The listing builds one solid part. Answer for the finished solid, in the listing's coordinates (mm). Coordinates: 2 decimals unless noted, no trailing zeros. Loops run counter-clockwise (first coordinate to the right, second up) from the corner with the lowest first, then second, coordinate; pieces in that order, holes last. Notation, with made-up numbers: (58, 81.5) -> (73, 81.5) arc R26 cw to (73, 107.5) -> close; hole circle Ø8 at (78, 74). An arc over 180 degrees is marked (long way). Answer in a Markdown table with one row per item.
```python
from build123d import *

# Parameters (mm, degrees)
SKETCH1_W           = 80
SKETCH1_H           = 80
SKETCH1_R           = 2
SKETCH1_R_2         = 1.75
BOSS_EXTRUDE1_DEPTH = 4
CUT_EXTRUDE2_DEPTH  = 57.709787515
FILLET1_R           = 10
FILLET2_R           = 20
BOSS_EXTRUDE3_DEPTH = 4
SKETCH6_R           = 1.75
CUT_EXTRUDE3_DEPTH  = 4
SKETCH7_R           = 1.5
CUT_EXTRUDE4_DEPTH  = 10
CHAMFER1_SIZE       = 8
CHAMFER1_SIZE2      = 11.425184054
SKETCH8_W           = 10
SKETCH8_H           = 34
BOSS_EXTRUDE4_DEPTH = 4
SKETCH9_R           = 2
CUT_EXTRUDE5_DEPTH  = 4
CHAMFER2_SIZE       = 10
CHAMFER2_SIZE2      = 8.390996312


with BuildPart() as part:
    # Sketch1 → Boss-Extrude1 (new body)
    with BuildSketch(Plane(origin=(0, 0, 0), x_dir=(1, 0, 0), z_dir=(0, 1, 0))):
        Rectangle(SKETCH1_W, SKETCH1_H)
        with Locations(Location((-24.748737342, 24.748737342, 0), (0, 0, 270))):
            Circle(SKETCH1_R, mode=Mode.SUBTRACT)
        with Locations(Location((24.748737342, 24.748737342, 0), (0, 0, 270))):
            Circle(SKETCH1_R, mode=Mode.SUBTRACT)
        with Locations(Location((24.748737342, -24.748737342, 0), (0, 0, 270))):
            Circle(SKETCH1_R, mode=Mode.SUBTRACT)
        with Locations(Location((-24.748737342, -24.748737342, 0), (0, 0, 270))):
            Circle(SKETCH1_R, mode=Mode.SUBTRACT)
        with Locations(Location((-10, 10, 0), (0, 0, 270))):
            Circle(SKETCH1_R_2, mode=Mode.SUBTRACT)
        with Locations(Location((10, 10, 0), (0, 0, 270))):
            Circle(SKETCH1_R_2, mode=Mode.SUBTRACT)
        with Locations(Location((10, -10, 0), (0, 0, 270))):
            Circle(SKETCH1_R_2, mode=Mode.SUBTRACT)
        with Locations(Location((-10, -10, 0), (0, 0, 270))):
            Circle(SKETCH1_R_2, mode=Mode.SUBTRACT)
        with Locations(Location((31.819805153, 31.819805153, 0), (0, 0, 270))):
            Circle(SKETCH1_R, mode=Mode.SUBTRACT)
        with Locations(Location((-31.819805153, 31.819805153, 0), (0, 0, 270))):
            Circle(SKETCH1_R, mode=Mode.SUBTRACT)
        with Locations(Location((-31.819805153, -31.819805153, 0), (0, 0, 270))):
            Circle(SKETCH1_R, mode=Mode.SUBTRACT)
        with Locations(Location((31.819805153, -31.819805153, 0), (0, 0, 270))):
            Circle(SKETCH1_R, mode=Mode.SUBTRACT)
    extrude(amount=BOSS_EXTRUDE1_DEPTH)

    # Sketch2 → Cut-Extrude2 (cut, through all)
    with BuildSketch(Plane(origin=(0, 4, 0), x_dir=(1, 0, 0), z_dir=(0, 1, 0))):
        Polygon((-40, 30), (-40, -30), (-17, -10), (-17, 10), align=None)
        Polygon((30, 40), (-30, 40), (-10, 17), (10, 17), align=None)
        Polygon((40, -30), (40, 30), (17, 10), (17, -10), align=None)
        Polygon((-30, -40), (30, -40), (10, -17), (-10, -17), align=None)
    extrude(amount=-CUT_EXTRUDE2_DEPTH, mode=Mode.SUBTRACT)

    # Fillet1
    # the kernel refuses this fillet: 10 mm, written as the material it takes off along each edge
    with BuildSketch(Plane(origin=(-30, 15.390762292, 40), x_dir=(-1, 0, 0), z_dir=(0, -1, 0)), Plane(origin=(-40, 15.390762292, 30), x_dir=(0.754605522163505, 0, -0.6561787149247863), z_dir=(0, -1, 0)), Plane(origin=(-40, 15.390762292, -30), x_dir=(0, 0, -1), z_dir=(0, -1, 0)), Plane(origin=(-30, 15.390762292, -40), x_dir=(0.6561787149247871, 0, 0.7546055221635043), z_dir=(0, -1, 0)), Plane(origin=(30, 15.390762292, -40), x_dir=(1, 0, 0), z_dir=(0, -1, 0)), Plane(origin=(40, 15.390762292, -30), x_dir=(-0.7546055221635045, 0, 0.6561787149247867), z_dir=(0, -1, 0)), Plane(origin=(40, 15.390762292, 30), x_dir=(0, 0, 1), z_dir=(0, -1, 0))) as fillet1_piece_1:
        with BuildLine():
            CenterArc((FILLET1_R * 0.455630491663, FILLET1_R), FILLET1_R, 221.009086902, 48.990913098)
            Line((-FILLET1_R * 0.2989750305, FILLET1_R * 0.343821285075), (0, 0))
            Line((0, 0), (FILLET1_R * 0.455630491663, 0))
        make_face()
    extrude(amount=26.781524583, mode=Mode.SUBTRACT)
    with BuildSketch(Plane(origin=(-40, -25, 40), x_dir=(0, 0, -1), z_dir=(0, 1, 0)), Plane(origin=(-40, -25, -40), x_dir=(1, 0, 0), z_dir=(0, 1, 0)), Plane(origin=(40, -25, -40), x_dir=(0, 0, 1), z_dir=(0, 1, 0)), Plane(origin=(40, -25, 40), x_dir=(-1, 0, 0), z_dir=(0, 1, 0))) as fillet1_piece_2:
        with BuildLine():
            CenterArc((FILLET1_R, -FILLET1_R), FILLET1_R, 90, 90)
            Line((0, -FILLET1_R), (0, 0))
            Line((0, 0), (FILLET1_R, 0))
        make_face()
    extrude(amount=54, mode=Mode.SUBTRACT)
    with BuildSketch(Plane(origin=(30, 15.390762292, 40), x_dir=(1, 0, 0), z_dir=(0, -1, 0))) as fillet1_piece_3:
        with BuildLine():
            CenterArc((FILLET1_R * 0.455630491663, -FILLET1_R), FILLET1_R, 90, 48.990913098)
            Line((-FILLET1_R * 0.2989750305, -FILLET1_R * 0.343821285075), (0, 0))
            Line((0, 0), (FILLET1_R * 0.455630491663, 0))
        make_face()
    extrude(amount=26.781524583, mode=Mode.SUBTRACT)

    # Fillet2
    fillet2_edges = [part.edges().sort_by_distance(p)[0] for p in [
        (10, 2, 17),
        (-10, 2, 17),
        (-17, 2, 10),
        (-17, 2, -10),
        (17, 2, -10),
        (17, 2, 10),
        (-10, 2, -17),
        (10, 2, -17),
    ]]
    fillet(fillet2_edges, radius=FILLET2_R)

    # Sketch5 → Boss-Extrude3 (add)
    with BuildSketch(Plane(origin=(0, 4, 0), x_dir=(1, 0, 0), z_dir=(0, 1, 0))):
        Polygon((-0.887390167, 17), (13.289046487, 12.123524967), (13.289046487, -13.496190448), (-0.887390167, -17), (59.112609833, -17), (59.112609833, 17), align=None)
    boss_extrude3 = extrude(amount=-BOSS_EXTRUDE3_DEPTH)

    # Sketch6 → Cut-Extrude3 (cut)
    with BuildSketch(Plane(origin=(0, 4, 0), x_dir=(1, 0, 0), z_dir=(0, 1, 0))):
        with Locations(Location((25, 10, 0), (0, 0, 270))):
            Circle(SKETCH6_R)
        with Locations(Location((45, 10, 0), (0, 0, 270))):
            Circle(SKETCH6_R)
        with Locations(Location((25, -10, 0), (0, 0, 270))):
            Circle(SKETCH6_R)
        with Locations(Location((45, -10, 0), (0, 0, 270))):
            Circle(SKETCH6_R)
    cut_extrude3 = extrude(amount=-CUT_EXTRUDE3_DEPTH, mode=Mode.SUBTRACT)

    # Mirror1: Boss-Extrude3, Cut-Extrude3 across plane
    add(boss_extrude3.mirror(Plane(origin=(0, 0, 0), x_dir=(0, 0, 1), z_dir=(1, 0, 0))))
    add(cut_extrude3.mirror(Plane(origin=(0, 0, 0), x_dir=(0, 0, 1), z_dir=(1, 0, 0))), mode=Mode.SUBTRACT)

    # Sketch7 → Cut-Extrude4 (cut)
    with BuildSketch(Plane(origin=(0, 4, 0), x_dir=(1, 0, 0), z_dir=(0, 1, 0))):
        with Locations(Location((55, 7.25, 0), (0, 0, 270))):
            Circle(SKETCH7_R)
        with Locations(Location((55, -7.25, 0), (0, 0, 270))):
            Circle(SKETCH7_R)
    extrude(amount=-CUT_EXTRUDE4_DEPTH, mode=Mode.SUBTRACT)

    # Chamfer1
    chamfer1_edges = [part.edges().sort_by_distance(p)[0] for p in [
        (59.112609833, 2, 17),
        (59.112609833, 2, -17),
    ]]
    chamfer1_side = [part.faces().sort_by_distance(p)[0] for p in [
        (59.112609833, 2, 0),
    ]]
    chamfer(chamfer1_edges, length=CHAMFER1_SIZE, length2=CHAMFER1_SIZE2, reference=chamfer1_side[0])

    # Sketch8 → Boss-Extrude4 (add)
    with BuildSketch(Plane(origin=(0, 4, 0), x_dir=(1, 0, 0), z_dir=(0, 1, 0))):
        with Locations((-64.112609833, 0)):
            Rectangle(SKETCH8_W, SKETCH8_H)
    extrude(amount=-BOSS_EXTRUDE4_DEPTH)

    # Sketch9 → Cut-Extrude5 (cut)
    with BuildSketch(Plane(origin=(0, 4, 0), x_dir=(1, 0, 0), z_dir=(0, 1, 0))):
        with Locations(Location((-64.112609833, 6, 0), (0, 0, 270))):
            Circle(SKETCH9_R)
        with Locations(Location((-64.112609833, -6, 0), (0, 0, 270))):
            Circle(SKETCH9_R)
        with Locations(Location((-59.112609833, -13, 0), (0, 0, 270))):
            Circle(SKETCH9_R)
        with Locations(Location((-59.112609833, 13, 0), (0, 0, 270))):
            Circle(SKETCH9_R)
    extrude(amount=-CUT_EXTRUDE5_DEPTH, mode=Mode.SUBTRACT)

    # Chamfer2
    chamfer2_edges = [part.edges().sort_by_distance(p)[0] for p in [
        (-69.112609833, 2, 17),
        (-69.112609833, 2, -17),
    ]]
    chamfer2_side = [part.faces().sort_by_distance(p)[0] for p in [
        (-69.112609833, 2, 0),
    ]]
    chamfer(chamfer2_edges, length=CHAMFER2_SIZE, length2=CHAMFER2_SIZE2, reference=chamfer2_side[0])


solid = part.part
```
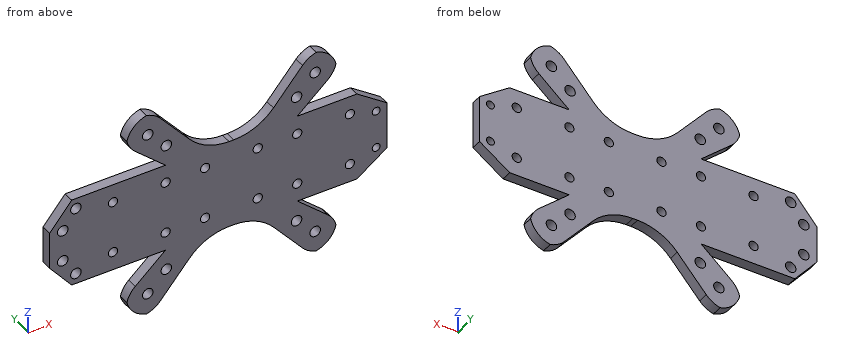
Item 1: Find the intervals of material crossed by probe 1 along Z at (x, y) = (-31, 3.3); probe 2 along Z at (x, y) = (-11.5, 2.4); probe 3 along X at (y, z) = (2.9, -6), in increasing order.
Findings below:
| item | result |
|---|---|
| probe 1 | z = -39.35 to -33.64, -30 to -22.17, -17 to 17, 22.17 to 30, 33.64 to 39.35 |
| probe 2 | z = -20.05 to -10.9, -9.1 to 9.1, 10.9 to 20.05 |
| probe 3 | x = -69.11 to -66.11, -62.11 to 54.17, 55.83 to 59.11 |
Item 2: Flat-ended cylindrical pins translate along their axes: pin 1 Ø1.4 at (x, y) = (-0.5, 2.5) entering from -Z; pin 2 Ø2 at (x, y) = (39.5, 2) entering from -Z; pin 3 Ø0.5 at (x, y) = (-0.5, 1.5) entering from +Z. Find the tip coordinate at first contact, or state that the pin passes through.
Findings below:
| item | result |
|---|---|
| pin 1 | stops at z = -17 |
| pin 2 | stops at z = -35.27 |
| pin 3 | stops at z = 17 |
Item 3: A cutting plane is placed at C-C, the plane x = 55. Determine the outline of the cut face in (y, z), plus the area to 3 significant figures.
Findings below:
| item | result |
|---|---|
| outline | (0, -11.88) -> (4, -11.88) -> (4, -8.75) -> (0, -8.75) -> close; (0, -5.75) -> (4, -5.75) -> (4, 5.75) -> (0, 5.75) -> close; (0, 8.75) -> (4, 8.75) -> (4, 11.88) -> (0, 11.88) -> close |
| area | 71.0 mm2 |
Item 4: A cutting plane is placed at D-D, the plane y = 1.55. Count the separate pieces of the cut face and the enclosed holes in it, plus the area to 3 significant figures.
Findings below:
| item | result |
|---|---|
| separate pieces | 1 |
| enclosed holes | 26 |
| area | 5,300 mm2 |
Item 5: A cutting plane is placed at B-B, the plane z = -13. Determine the outline of the cut face in (x, y).
Findings below:
| item | result |
|---|---|
| outline | (-64.08, 0) -> (-61.11, 0) -> (-61.11, 4) -> (-64.08, 4) -> close; (-57.11, 0) -> (53.4, 0) -> (53.4, 4) -> (-57.11, 4) -> close |
Item 6: A cutting plane is placed at A-A, the plane x = -45. Determine the outline of the cut face in (y, z).
Findings below:
| item | result |
|---|---|
| outline | (0, -17) -> (4, -17) -> (4, -11.75) -> (0, -11.75) -> close; (0, -8.25) -> (4, -8.25) -> (4, 8.25) -> (0, 8.25) -> close; (0, 11.75) -> (4, 11.75) -> (4, 17) -> (0, 17) -> close |
